Geometry check sheet. Reference: the model listing, model coordinates, mm. Round coordinates to 2 decimals unless told otherwise and drop trailing zeros. Order: outer loops, then holes, each group sorted by start corner. A loop starts at its lowest first (then second) coordinate and runs counter-clockwise, first axis right, second up. Notation, with made-up numbers: (12.25, -22) -> (47.25, -22) arc R24 ccw to (47.25, 17) -> close; hole circle Ø7 at (26, 45.25). An arc over 180 degrees is marked (long way). Use a Markdown table: item, result. Add a question column.
Item 1: Sectioned sample at A-A, the plane z = 0.3. Record the cut outline in (x, y), and give its area (3 significant figures).
Item 2: Material ranges on probe 1 along X at (y, z) = (2.5, 0.3); probe 2 along Y at (x, z) = (3, 0.1), recorded low to high. Write a range as [from, to].
Item 3: Sectioned sample at C-C, the plane y = 1.25. Record the cut outline in (x, z).
Item 4: Mould release check, pull along Y, two halves, no side actions. Record for faces 1 (the cylindrical face through (0.1, -3, 0.2)), 2 (the flat face through (0, 0, 0.5)), 3 (the cylindrical face through (0.23, 2.99, 0.25)): pulls with the +Y half, pulls with the -Y half, needs draft (parallel to the pull), parting line crosses it, or undercut.
Item 5: Sectioned sample at B-B, the plane x = -2.75. Record the cut outline in (y, z).
from build123d import *

# Parameters (mm, degrees)
F1_DEPTH = 0.5
F2_R     = 0.4


with BuildPart() as f1:
    # F0 (on Top) → F1 (new body)
    with BuildSketch(Plane.XY):
        with BuildLine():
            Line((-4.062, 0.861426), (-2.873664, 0.861426))
            ThreePointArc((-2.873664, 0.861426), (-3, 0), (-2.873664, -0.861426))
            Line((-2.873664, -0.861426), (-4.062, -0.861426))
            Line((-4.062, -0.861426), (-4.062, -1.461426))
            Line((-4.062, -1.461426), (-2.619968, -1.461426))
            ThreePointArc((-2.619968, -1.461426), (0.225595, -2.991506), (2.809509, -1.051979))
            Line((2.809509, -1.051979), (4.013425, 0))
            Line((4.013425, 0), (2.809509, 1.051979))
            ThreePointArc((2.809509, 1.051979), (0.225595, 2.991506), (-2.619968, 1.461426))
            Line((-2.619968, 1.461426), (-4.062, 1.461426))
            Line((-4.062, 1.461426), (-4.062, 0.861426))
        make_face()
    extrude(amount=F1_DEPTH)

    # F2
    f2_edges = [f1.edges().sort_by_distance(p)[0] for p in [
        (4.013425, 0, 0.25),
        (2.809509, 1.051979, 0.25),
        (2.809509, -1.051979, 0.25),
    ]]
    fillet(f2_edges, radius=F2_R)


solid = f1.part
Found:
| question | item | result |
|---|---|---|
| 1 | outline | (-4.06, -1.46) -> (-2.62, -1.46) arc R3 ccw to (2.78, -1.14) arc R0.4 cw to (2.88, -0.99) -> (3.67, -0.3) arc R0.4 ccw to (3.67, 0.3) -> (2.88, 0.99) arc R0.4 cw to (2.78, 1.14) arc R3 ccw to (-2.62, 1.46) -> (-4.06, 1.46) -> (-4.06, 0.86) -> (-2.87, 0.86) arc R3 ccw to (-2.87, -0.86) -> (-4.06, -0.86) -> close |
| 1 | area | 30.8 mm2 |
| 2 | probe 1 | x = [-1.66, 1.66] |
| 2 | probe 2 | y = [-0.89, 0.89] |
| 3 | outline | (-4.06, 0) -> (2.73, 0) -> (2.73, 0.5) -> (-4.06, 0.5) -> close |
| 4 | face 1 | pulls with the -Y half |
| 4 | face 2 | needs draft |
| 4 | face 3 | pulls with the +Y half |
| 5 | outline | (-1.46, 0) -> (1.46, 0) -> (1.46, 0.5) -> (-1.46, 0.5) -> close |
